```python
from build123d import *

# Parameters (mm, degrees)
SKETCH1_W           = 43.25
SKETCH1_H           = 50.9
BOSS_EXTRUDE1_DEPTH = 1.56
FILLET1_R           = 3
FILLET2_R           = 3
SKETCH2_R           = 1.5875
CUT_EXTRUDE1_DEPTH  = 1.56


with BuildPart() as part:
    # Sketch1 → Boss-Extrude1 (new body)
    with BuildSketch(Plane(origin=(0, 0, 0), x_dir=(1, 0, 0), z_dir=(0, 1, 0))):
        Rectangle(SKETCH1_W, SKETCH1_H)
    extrude(amount=BOSS_EXTRUDE1_DEPTH)

    # Fillet1
    fillet1_edges = [part.edges().sort_by_distance(p)[0] for p in [
        (21.625, 0.78, 25.45),
    ]]
    fillet(fillet1_edges, radius=FILLET1_R)

    # Fillet2
    fillet2_edges = [part.edges().sort_by_distance(p)[0] for p in [
        (-21.625, 0.78, -25.45),
        (21.625, 0.78, -25.45),
        (-21.625, 0.78, 25.45),
    ]]
    fillet(fillet2_edges, radius=FILLET2_R)

    # Sketch2 → Cut-Extrude1 (cut)
    with BuildSketch(Plane(origin=(0, 1.56, 0), x_dir=(1, 0, 0), z_dir=(0, 1, 0))):
        with Locations(Location((-17.805, 0, 0), (0, 0, 270))):
            Circle(SKETCH2_R)
        with Locations(Location((17.805, 0, 0), (0, 0, 270))):
            Circle(SKETCH2_R)
    extrude(amount=-CUT_EXTRUDE1_DEPTH, mode=Mode.SUBTRACT)


solid = part.part
```
Part model, mm, in its own coordinate system. Give positions to 0.01 mm unless a question says otherwise; leave off trailing zeros. Write each loop counter-clockwise with the first axis right and the second up, starting at its lowest first coordinate (ties: lowest second). Pieces come first, ordered by that corner, then holes. Notation, with made-up numbers: (28.25, -1) -> (40.25, -1) arc R29 ccw to (40.25, 22) -> close; hole circle Ø5 at (67, 48). An arc over 180 degrees is marked (long way). Put each result on its own line as item: value. Start each with the question number.
Item 1: Wall check: L1, parallel to X at y = 1, z = 0 (1 decimal); L2, parallel to Z at x = 18.5, y = 0.1; L3, parallel to X at y = 0.65, z = 1 (3 decimals). Give the ranges that are in metal, low to high. Write a range as [from, to].
Item 2: Pin check, flat tip, straight feed: pin 1 Ø1.9 at (x, z) = (17.805, 0) entering from +Y. Stop position of the tip, or through.
Item 3: Pull direction Z, two halves, no side cores. Call faces 1 (the face through (-20.77, 0.79, -24.55)), 2 (the face through (21.625, 1, 0)), 3 (the face through (20.723, 0.791, 24.595)), 4 (the face through (-19.355, 0.791, -0.344)): pulls with the +Z half, pulls with the -Z half, needs draft (parallel to the pull), parting line crosses it, or undercut.
Item 4: Cut at A-A (z = 0). List the corners of the cut face in (x, y) (1 decimal), then the cut area to 3 significant figures.
Answer list:
1. L1: x = [-21.6, -19.4], [-16.2, 16.2], [19.4, 21.6]
1. L2: z = [-25.45, -1.43], [1.43, 25.45]
1. L3: x = [-21.625, -19.038], [-16.572, 16.572], [19.038, 21.625]
2. pin 1: passes through
3. face 1: pulls with the -Z half
3. face 2: needs draft
3. face 3: pulls with the +Z half
3. face 4: undercut
4. outline: (-21.6, 0) -> (-19.4, 0) -> (-19.4, 1.6) -> (-21.6, 1.6) -> close; (-16.2, 0) -> (16.2, 0) -> (16.2, 1.6) -> (-16.2, 1.6) -> close; (19.4, 0) -> (21.6, 0) -> (21.6, 1.6) -> (19.4, 1.6) -> close
4. area: 57.6 mm2
